Read the model definition and answer for the solid it produces. Units are mm, in the model's axes. Coordinates: 2 decimals unless noted, no trailing zeros. Loops run counter-clockwise (first coordinate to the right, second up) from the corner with the lowest first, then second, coordinate; pieces in that order, holes last. Notation, with made-up numbers: M 51,49 L 61,49 A32 cw 61,82 Z; hole C 38.5,2 d8. An arc over 180 degrees is marked long. Use one line per item in the form item = value. Start each with the question number.
1. Find the intervals of material crossed by probe 1 along X at (y, z) = (72.5, 8.25); probe 2 along Y at (x, z) = (6, 5.5); probe 3 along X at (y, z) = (-55.5, 3), in increasing order. Write a range as [from, to].
2. Flat-ended cylindrical pins translate along their axes: pin 1 (1 mm diameter, centred on y = 117, z = 3, fed in from +X); pin 2 (1.8 mm diameter, centred on y = -54.5, z = 7, fed in from +X); pin 3 (3 mm diameter, centred on x = 18, y = -30.5, fed in from +Z); pin 4 (2 mm diameter, centred on y = 23.5, z = 5, fed in from -X). Find the tip coordinate at first contact, or state that the pin passes through.
3. The part is cut by section B-B (x = -10). Give the vertices of the cut face in (y, z).
4. The part is cut by section A-A (y = 43). Give the vertices of the cut face in (x, z).
from build123d import *

# Parameters (mm, degrees)
EXTRUDE_1_DEPTH = 10


with BuildPart() as part:
    # Эскиз1 → Бобышка-Вытянуть1 (new body)
    with BuildSketch(Plane.XY):
        Polygon((-53.85138596, 14.018578311), (-57.04541686, 22.64246174), (-51.296161241, 27.114105), (-42.672277811, 20.40664011), (-42.672277811, 27.114105), (-31.732721979, 27.114105), (-61.19765703, 47.236499669), (-65.092910636, 57.753684406), (-65.092910636, 73.746956137), (-63.145283833, 88.758901366), (-54.17078905, 101.900125869), (-43.667374626, 115.404515844), (-26.130435815, 129.044357141), (-5.466398977, 136.697704118), (16.417293835, 139.224589583), (37.817300864, 139.224589583), (57.620292443, 132.871030629), (78.381493292, 122.224436492), (94.189290443, 101.900125869), (101.836400486, 81.252928751), (101.836400486, 65.750320271), (94.189290443, 55.918321644), (84.798214398, 48.614151387), (86.452679963, 34.285913445), (89.49375242, 34.637062671), (92.132772709, 31.244036586), (98.012845465, 35.817426507), (104.233890809, 15.685456171), (98.619402154, 4.737022793), (100.083204907, 0), (100.083204907, -10.326628952), (100.083204907, -18.075202764), (92.132772709, -28.297187018), (93.303752164, -38.438269801), (89.436859181, -43.40998935), (86.452679963, -41.088961069), (83.206856787, -30.585128953), (80.338686983, -34.272775844), (82.444978452, -41.088961069), (82.444978452, -46.241720155), (76.912286554, -46.241720155), (76.912286554, -41.088961069), (68.000892867, -41.088961069), (63.619059508, -37.680868456), (62.211127726, -48.532944823), (59.324618186, -52.244171373), (59.324618186, -55.882780265), (62.915093617, -65.577063928), (62.915093617, -69.038718479), (59.324618186, -69.038718479), (57.099268832, -67.307891203), (50.877031559, -54.063475819), (46.532092284, -57.442873034), (36.394456911, -52.244171373), (25.513596442, -38.254493627), (25.513596442, -34.272775844), (18.873446088, -25.735439675), (14.495397156, -34.272775844), (8.866486546, -45.2493325), (7.182610552, -48.532944823), (2.172454709, -50.388558098), (7.182610552, -57.442873034), (9.485737931, -60.685683511), (9.485737931, -65.577063928), (7.182610552, -65.577063928), (0, -61.893734627), (-1.648467257, -57.442873034), (-4.261176492, -50.388558098), (-7.199449567, -50.388558098), (-12.097138316, -50.388558098), (-15.798417396, -50.388558098), (-20.970033483, -43.10690664), (-26.130435815, -40.460590099), (-29.111221424, -36.263634735), (-34.898905221, -28.114558035), (-34.898905221, -23.186194891), (-37.202499895, -19.942726459), (-47.699218285, -5.163314476), (-47.699218285, -2.378627093), align=None)
    extrude(amount=EXTRUDE_1_DEPTH)


solid = part.part
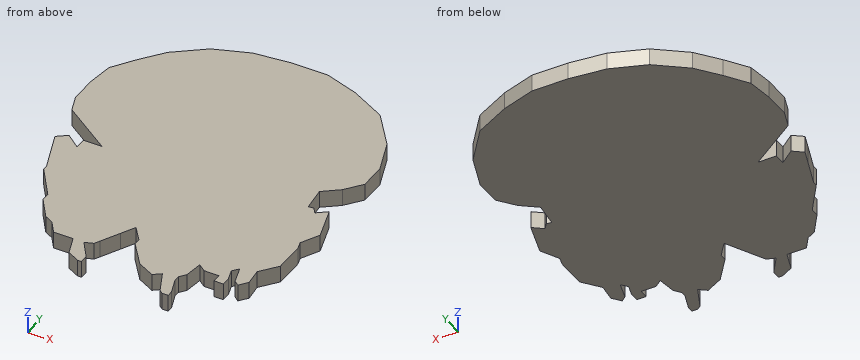
Computed values:
q1.probe_1 = [-65.09, 101.84]
q1.probe_2 = [-64.97, -55.78], [-48.97, 138.02]
q1.probe_3 = [-2.37, 5.8], [42.74, 49.03], [51.55, 59.32]
q2.pin_1 = 82.83
q2.pin_2 = 59.32
q2.pin_3 = 10
q2.pin_4 = -57.05
q3.outline = M -50.39,0 L 135.02,0 L 135.02,10 L -50.39,10 Z
q4.outline = M -54.99,0 L 85.45,0 L 85.45,10 L -54.99,10 Z
